```python
from build123d import *

# Parameters (mm, degrees)
BOSS_EXTRUDE1_DEPTH   = 2.54
F_8_CLEARANCE_HOLE1_D = 4.4958
F_4_CLEARANCE_HOLE1_D = 3.2639


with BuildPart() as part:
    # Sketch1 → Boss-Extrude1 (new body)
    with BuildSketch(Plane.XY):
        with BuildLine():
            Line((0.254, -5.073646026), (25.5905, -3.80523452))
            ThreePointArc((25.5905, -3.80523452), (29.21, 0), (25.5905, 3.80523452))
            Line((25.5905, 3.80523452), (0.254, 5.073646026))
            ThreePointArc((0.254, 5.073646026), (-5.08, 0), (0.254, -5.073646026))
        make_face()
    extrude(amount=BOSS_EXTRUDE1_DEPTH)

    # #8 Clearance Hole1 (through all)
    with Locations(Plane.XY.offset(2.54)):
        with Locations((0, 0)):
            Hole(F_8_CLEARANCE_HOLE1_D / 2)

    # #4 Clearance Hole1 (through all)
    with Locations(Plane(origin=(25.4, 0, 2.54), x_dir=(1, 0, 0), z_dir=(0, 0, 1))):
        with Locations((0, 0)):
            Hole(F_4_CLEARANCE_HOLE1_D / 2)


solid = part.part
```
Part model, mm, in its own coordinate system. Coordinates: 2 decimals unless noted, no trailing zeros. Order: outer loops, then holes, each group sorted by start corner. A loop starts at its lowest first (then second) coordinate and runs counter-clockwise, first axis right, second up. Notation, with made-up numbers: (8, 39.5) -> (50, 39.5) arc R29 ccw to (50, 69.5) -> close; hole circle Ø2 at (-20.75, 54.5). An arc over 180 degrees is marked (long way). Put each result on its own line as item: value. Start each with the question number.
(1) Band-saw the part on D-D (x = 21). Give the cut face in (y, z).
(2) Mould opens along X. For faces 1 (the face through (-2.076, -0.861, 1.252)), 2 (the face through (29.21, -0.08, 1.25)), 3 (the face through (12, 0, 2.54)) say: pulls with the +X half, pulls with the -X half, needs draft (parallel to the pull), parting line crosses it, or undercut.
(3) Probe line 1 along Y through (x, z) = (25.5, 2.25); line 2 along X through (y, z) = (1.25, 1.45); line 3 along Y through (x, z) = (0, 1.55). List the from-to ranges inside material, lowest first. Write a range as [from, to].
(4) Pin check, flat tips, straight feed: pin 1 Ø1.5 at (x, z) = (25.5, 1.5) entering from +Y; pin 2 Ø1 at (x, z) = (15.5, 1.5) entering from +Y. Stop position of each tip, or through.
(5) Band-saw the part on B-B (x = 26). Give the cut face in (y, z), then the cut area to 3 significant figures.
(6) Band-saw the part on A-A (y = 0). Give the cut face in (x, z), then the cut area to 3 significant figures.
Determined:
1. outline: (-4.04, 0) -> (4.04, 0) -> (4.04, 2.54) -> (-4.04, 2.54) -> close
2. face 1: undercut
2. face 2: pulls with the +X half
2. face 3: needs draft
3. line 1: y = [-3.81, -1.63], [1.63, 3.81]
3. line 2: x = [-4.92, -1.87], [1.87, 24.35], [26.45, 29]
3. line 3: y = [-5.08, -2.25], [2.25, 5.08]
4. pin 1: stops at y = 3.85
4. pin 2: stops at y = 4.34
5. outline: (-3.76, 0) -> (-1.52, 0) -> (-1.52, 2.54) -> (-3.76, 2.54) -> close; (1.52, 0) -> (3.76, 0) -> (3.76, 2.54) -> (1.52, 2.54) -> close
5. area: 11.4 mm²
6. outline: (-5.08, 0) -> (-2.25, 0) -> (-2.25, 2.54) -> (-5.08, 2.54) -> close; (2.25, 0) -> (23.77, 0) -> (23.77, 2.54) -> (2.25, 2.54) -> close; (27.03, 0) -> (29.21, 0) -> (29.21, 2.54) -> (27.03, 2.54) -> close
6. area: 67.4 mm²
